from build123d import *

# Parameters (mm, degrees)
BOSS_EXTRUDE1_DEPTH = 3.175
FILLET1_R           = 2.54
FILLET2_R           = 6.35
SKETCH2_R           = 2.032
CUT_EXTRUDE1_DEPTH  = 116.785553087


with BuildPart() as part:
    # Sketch1 → Boss-Extrude1 (new body)
    with BuildSketch(Plane.XY):
        with BuildLine():
            Line((0, 0), (0, 106.872811366))
            Line((0, 106.872811366), (-40.80699964, 33.868121814))
            ThreePointArc((-40.80699964, 33.868121814), (-60.999593642, 11.461483708), (-88.9, 0))
            Line((-88.9, 0), (0, 0))
        make_face()
    extrude(amount=BOSS_EXTRUDE1_DEPTH)

    # Fillet1
    fillet1_edges = [part.edges().sort_by_distance(p)[0] for p in [
        (-88.9, 0, 1.5875),
    ]]
    fillet(fillet1_edges, radius=FILLET1_R)

    # Fillet2
    fillet2_edges = [part.edges().sort_by_distance(p)[0] for p in [
        (0, 106.872811366, 1.5875),
        (0, 0, 1.5875),
    ]]
    fillet(fillet2_edges, radius=FILLET2_R)

    # Sketch2 → Cut-Extrude1 (cut, through all)
    with BuildSketch(Plane.XY.offset(3.175)):
        with Locations((-6.35, 6.35)):
            Circle(SKETCH2_R)
        with Locations((-6.35, 82.497944882)):
            Circle(SKETCH2_R)
    extrude(amount=-CUT_EXTRUDE1_DEPTH, mode=Mode.SUBTRACT)


solid = part.part
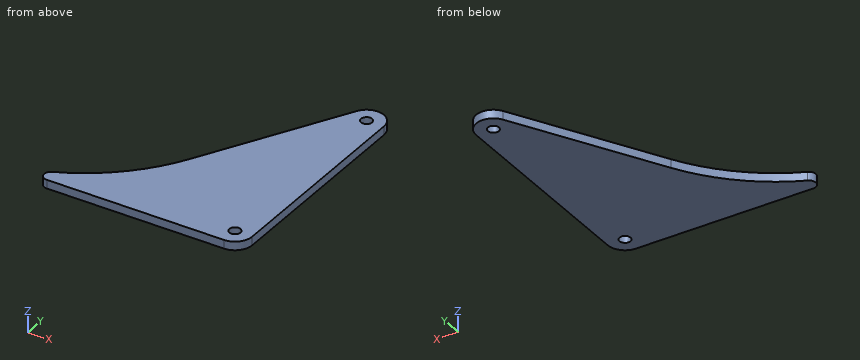
Source: CAD feature listing. Evaluate the final solid. Frame: model axes, mm. Give positions to 0.01 mm unless a question says otherwise; leave off trailing zeros. Write each loop counter-clockwise with the first axis right and the second up, starting at its lowest first coordinate (ties: lowest second). Pieces come first, ordered by that corner, then holes. Notation, with made-up numbers: M -23.5,62 L 19.5,62 A3 ccw 19.5,67 Z; hole C -13.5,34 d4. An arc over 180 degrees is marked long. Return JSON: item names as keys, results as strings. Group by question number.
1) Cut plane B-B, the plane x = -49. Output: boundary loops of the cut face in (y, z) (3 decimals), plus the area to 3 significant figures.
2) Cut plane C-C, the plane y = 42. Output: boundary loops of the cut face in (x, z) (3 decimals).
3) Material intervals for line 1 along X through (y, z) = (81, 0.6); line 2 along X through (y, z) = (84, 2.3); line 3 along Y through (x, z) = (-11.5, 1.8), sorted ascending. Write a range as [from, to].
4) Cut plane A-A, the plane z = 1.9. Output: boundary loops of the cut face in (x, y).
Recorded:
{
 "1": {"outline": "M 0,0 L 22.256,0 L 22.256,3.175 L 0,3.175 Z", "area": "70.7 mm²"},
 "2": {"outline": "M -36.262,0 L 0,0 L 0,3.175 L -36.262,3.175 Z"},
 "3": {"line 1": "x = [-14.46, -7.72], [-4.98, 0]", "line 2": "x = [-12.79, -7.72], [-4.98, -0.18]", "line 3": "y = [0, 86.21]"},
 "4": {"outline": "M -72.66,4.86 A2.54 ccw -71.64,0 L -6.35,0 A6.35 ccw 0,6.35 L 0,82.5 A6.35 ccw -11.89,85.6 L -40.81,33.87 A67.96 cw Z; hole C -6.35,6.35 d4.06; hole C -6.35,82.5 d4.06"}
}
